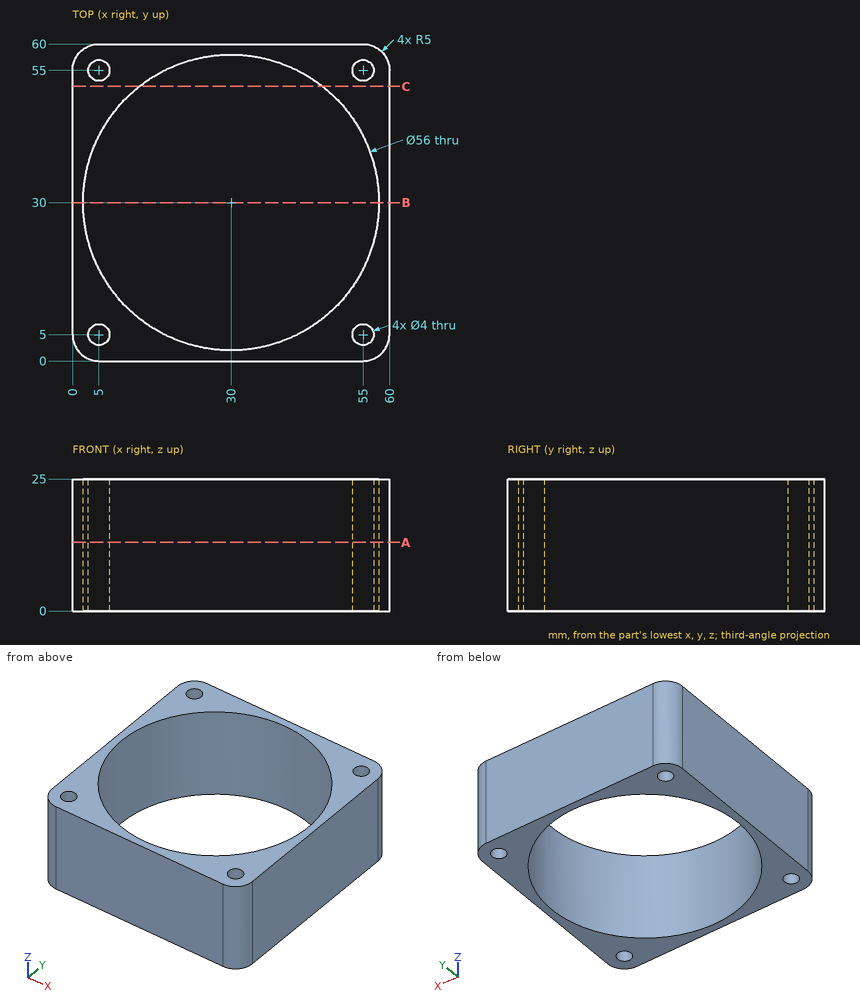
Source: three-view drawing plus pictorial views. Frame: mm from the lowest corner of the part. Give positions to 0.01 mm unless a question says otherwise; leave off trailing zeros. Order: outer loops, then holes, each group sorted by start corner. A loop starts at its lowest first (then second) coordinate and runs counter-clockwise, first axis right, second up.
1. Section A-A on z = 13. Return the cut outline in (x, y).
Derived:
outline: (0, 5) arc R5 ccw to (5, 0) - (55, 0) arc R5 ccw to (60, 5) - (60, 55) arc R5 ccw to (55, 60) - (5, 60) arc R5 ccw to (0, 55) - close; hole circle Ø56 at (30, 30); hole circle Ø4 at (5, 5); hole circle Ø4 at (5, 55); hole circle Ø4 at (55, 5); hole circle Ø4 at (55, 55)
2. Section B-B on y = 30. Return the cut outline in (x, z), and give its area (3 significant figures).
Derived:
outline: (0, 0) - (2, 0) - (2, 25) - (0, 25) - close; (58, 0) - (60, 0) - (60, 25) - (58, 25) - close
area: 100 mm2
3. Pin query (flat end, axial travel): pin 1 (3 mm diameter, centred on x = 5, y = 55, fed in from +Z). Return the tip coordinate at first contact, or that it passes through.
Derived:
pin 1: passes through
4. Material intervals for L1, parallel to Y at x = 5, z = 16.25; L2, parallel to Y at x = 30, z = 12.5; L3, parallel to Y at x = 54, z = 8.75, sorted ascending.
Derived:
L1: y = 0 to 3, 7 to 17.39, 42.61 to 53, 57 to 60
L2: y = 0 to 2, 58 to 60
L3: y = 0 to 3.27, 6.73 to 15.58, 44.42 to 53.27, 56.73 to 60
5. Section C-C on y = 52. Return the cut outline in (x, z), and give its area (3 significant figures).
Derived:
outline: (0, 0) - (12.68, 0) - (12.68, 25) - (0, 25) - close; (47.32, 0) - (60, 0) - (60, 25) - (47.32, 25) - close
area: 634 mm2
